Read the model definition and answer for the solid it produces. Units are mm, in the model's axes. A direction names the side the tool comes from. Coordinates: 2 decimals unless noted, no trailing zeros. Loops run counter-clockwise (first coordinate to the right, second up) from the corner with the lowest first, then second, coordinate; pieces in that order, holes last. Notation, with made-up numbers: M 54,-1 L 68,-1 A30 cw 68,38 Z; hole C 77,35 d11. An arc over 180 degrees is marked long. One line per item, written item: value. Start each with the question number.
```python
from build123d import *

# Parameters (mm, degrees)
F0_W     = 100
F0_H     = 50
F1_DEPTH = 25
F2_W     = 10
F2_H     = 10
F3_DEPTH = 15
F4_DEPTH = 18
F5_SCALE = 0.1


with BuildPart() as f1:
    # F0 (on Front) → F1 (new body)
    with BuildSketch(Plane.XZ):
        with Locations((-18.9008015549, 25)):
            Rectangle(F0_W, F0_H)
    extrude(amount=F1_DEPTH)

    # F2 (on face) → F3 (join)
    with BuildSketch(Plane.XZ.offset(25)):
        with Locations((-63.9008015549, 5)):
            Rectangle(F2_W, F2_H)
        with Locations((-63.9008015549, 45)):
            Rectangle(F2_W, F2_H)
        with Locations((26.0991984451, 45)):
            Rectangle(F2_W, F2_H)
        with Locations((26.0991984451, 5)):
            Rectangle(F2_W, F2_H)
    extrude(amount=F3_DEPTH)

    # F4 (cut): a face of the model
    f4_faces = [f1.faces().sort_by_distance(p)[0] for p in [
        (-18.9008015549, -25, 25),
    ]]
    extrude(f4_faces, amount=-F4_DEPTH, mode=Mode.SUBTRACT)


with BuildPart() as f1_1:
    # F5: moved
    add(f1.part.scale(F5_SCALE))


solid = f1_1.part
```
1) Section D-D (z = 1.3) is taken. Determine the outline of the cut face in (x, y), then the cut area to 3 significant figures.
2) A tool of negligible diameter and unlimited length cuts with its end or side. For faces 4 (the face through (-6.4, -2.3, 4)), 5 (the face through (-5.89, -2.4, 0.5)), 6 (the face through (-6.4, -4, 0.5)), from which of +Z, -Z, +X, -X, +Y, -Y can it reach the whole face along a straight path? Write none if from no direction.
3) Section A-A (y = -1.1) is taken. Determine the outline of the cut face in (x, z).
4) A flat-ended cylindrical pin translates along its axis: pin 1 (1.5 mm diameter, centred on x = -4, z = 3.5, fed in from -Y). Find the tip coordinate at first contact, or state that the pin passes through.
5) For a pull along X with two mould halves and no side action, classify faces 1 (the face through (2.11, -2.3, 4.5)), 2 (the face through (2.6, -4, 4.5)), 3 (the face through (-6.89, -0.2, 2.5)) as released by +X, released by -X, zero draft, split by the parting line, or undercut.
6) Section C-C (x = -4.5) is taken. Determine the outline of the cut face in (y, z).
7) Section B-B (z = 0.6) is taken. Determine the outline of the cut face in (x, y), then the cut area to 3 significant figures.
8) Consider line 1 along X through (y, z) = (-2.7, 4.1); line 2 along Y through (x, z) = (0, 4.7). Determine where each line is inside the solid, lowest interval first.
Results found:
1. outline: M -6.89,-0.7 L 3.11,-0.7 L 3.11,0 L -6.89,0 Z
1. area: 7.00 mm²
2. face 4: +X, -X, -Y
2. face 5: +Z, -Z, -Y
2. face 6: +Z, -Z, +X, -X, -Y
3. outline: M -6.89,0 L -5.89,0 L -5.89,1 L -6.89,1 Z; M -6.89,4 L -5.89,4 L -5.89,5 L -6.89,5 Z; M 2.11,0 L 3.11,0 L 3.11,1 L 2.11,1 Z; M 2.11,4 L 3.11,4 L 3.11,5 L 2.11,5 Z
4. pin 1: stops at y = -0.7
5. face 1: undercut
5. face 2: zero draft
5. face 3: released by -X
6. outline: M -0.7,0 L 0,0 L 0,5 L -0.7,5 Z
7. outline: M -6.89,-4 L -5.89,-4 L -5.89,-0.7 L 2.11,-0.7 L 2.11,-4 L 3.11,-4 L 3.11,0 L -6.89,0 Z
7. area: 13.6 mm²
8. line 1: x = -6.89 to -5.89, 2.11 to 3.11
8. line 2: y = -0.7 to 0
